```python
from build123d import *

# Parameters (mm, degrees)
F1_DEPTH = 18
F2_R     = 4
F3_DEPTH = 14


with BuildPart() as f1:
    # F0 (on Front) → F1 (new body)
    with BuildSketch(Plane.XZ):
        Polygon((355.5, 202), (-355.5, 202), (-355.5, 177), (-337.5, 177), (-337.5, 127), (-355.5, 127), (-355.5, 77), (-337.5, 77), (-337.5, 27), (-355.5, 27), (-355.5, -23), (-337.5, -23), (-337.5, -73), (-355.5, -73), (-355.5, -123), (-337.5, -123), (-337.5, -173), (-355.5, -173), (-355.5, -198), (355.5, -198), (355.5, -173), (337.5, -173), (337.5, -123), (355.5, -123), (355.5, -73), (337.5, -73), (337.5, -23), (355.5, -23), (355.5, 27), (337.5, 27), (337.5, 77), (355.5, 77), (355.5, 127), (337.5, 127), (337.5, 177), (355.5, 177), align=None)
    extrude(amount=F1_DEPTH)

    # F2 (on face) → F3 (cut)
    with BuildSketch(Plane.XZ.offset(18)):
        with Locations((-155.5, -118)):
            Circle(F2_R)
        with Locations((-155.5, 122)):
            Circle(F2_R)
    extrude(amount=-F3_DEPTH, mode=Mode.SUBTRACT)


solid = f1.part
```
Could you check a few things on this model? Use its own coordinates, in mm. A direction names the side the tool comes from. Give positions to 0.01 mm unless a question says otherwise; leave off trailing zeros. Loops run counter-clockwise (first coordinate to the right, second up) from the corner with the lowest first, then second, coordinate; pieces in that order, holes last. Notation, with made-up numbers: (17, 21) -> (63, 21) arc R17 cw to (63, 35) -> close; hole circle Ø2 at (31, 80). An arc over 180 degrees is marked (long way). Put each result on its own line as item: value.
(1) Thinking about a two-plate mould opening in Z: for faces 4 (the face through (347, -9, 27)), 5 (the face through (5, -9, 202)), 6 (the face through (-5, -9, -198)), which applies, pulls with the +Z half, pulls with the -Z half, needs draft (parallel to the pull), parting line crosses it, or undercut?
Computed:
face 4: undercut
face 5: pulls with the +Z half
face 6: pulls with the -Z half
(2) For faces 1 (the face through (-337.5, -9, -48)), 2 (the face through (-355.5, -9, 2)), 3 (the face through (347, -9, -73)), which set-ups out of +Z, -Z, +X, -X, +Y, -Y let a thin tool reach every point of the face, with its end or its side?
Computed:
face 1: -X, +Y, -Y
face 2: +Z, -Z, -X, +Y, -Y
face 3: +X, +Y, -Y
(3) I'm going to push flat-ended pins straight in: pin 1 Ø9 at (y, z) = (-6, -144) entering from -X; pin 2 Ø4 at (x, z) = (-155.5, 123.5) entering from -Y. Where does each tip first touch, or does it pass through?
Computed:
pin 1: x = -337.5
pin 2: y = -4
(4) Imagine slicing it at A-A on z = 139.5. Write out the boundary of the cut face in (x, y), plus the area to 4 significant figures.
Computed:
outline: (-337.5, -18) -> (337.5, -18) -> (337.5, 0) -> (-337.5, 0) -> close
area: 12,150 mm^2
(5) Please list where these lines run through material, in increasing order: probe 1 along Z at (x, y) = (-155.5, -9); probe 2 along X at (y, z) = (-10.75, -131). Write a range as [from, to].
Computed:
probe 1: [-198, -122], [-114, 118], [126, 202]
probe 2: [-337.5, 337.5]
(6) Imagine slicing it at B-B on y = -12.25. State how many separate pieces and enclosed holes the cut face has, plus the area to 3 significant figures.
Computed:
separate pieces: 1
enclosed holes: 2
area: 277,000 mm^2
